from build123d import *

# Parameters (mm, degrees)
SKETCH1_R           = 2.5527
BOSS_EXTRUDE1_DEPTH = 2.54
SKETCH7_W           = 88.9
SKETCH7_H           = 19.05
BOSS_EXTRUDE2_DEPTH = 2.54
SKETCH6_W           = 38.1
SKETCH6_H           = 2.54
SKETCH6_W_2         = 2.54
SKETCH6_H_2         = 12.7
BOSS_EXTRUDE3_DEPTH = 16.51
CUT_EXTRUDE1_DEPTH  = 3.54


with BuildPart() as part:
    # Sketch1 → Boss-Extrude1 (new body)
    with BuildSketch(Plane(origin=(0, 0, 0), x_dir=(1, 0, 0), z_dir=(0, 1, 0))):
        with BuildLine():
            Line((44.45, -20.3835), (-44.45, -20.3835))
            Line((-44.45, -20.3835), (-44.45, 20.3835))
            Line((-44.45, 20.3835), (-35.2425, 20.3835))
            ThreePointArc((-35.2425, 20.3835), (-32.99743597, 19.45356403), (-32.0675, 17.2085))
            Line((-32.0675, 17.2085), (-32.0675, 1.3335))
            Line((-32.0675, 1.3335), (32.0675, 1.3335))
            Line((32.0675, 1.3335), (32.0675, 17.2085))
            ThreePointArc((32.0675, 17.2085), (32.99743597, 19.45356403), (35.2425, 20.3835))
            Line((35.2425, 20.3835), (44.45, 20.3835))
            Line((44.45, 20.3835), (44.45, -20.3835))
        make_face()
        with Locations((37.1475, -14.0335)):
            Circle(SKETCH1_R, mode=Mode.SUBTRACT)
        with Locations((37.1475, 14.0335)):
            Circle(SKETCH1_R, mode=Mode.SUBTRACT)
        with Locations((-37.1475, -14.0335)):
            Circle(SKETCH1_R, mode=Mode.SUBTRACT)
        with Locations((-37.1475, 14.0335)):
            Circle(SKETCH1_R, mode=Mode.SUBTRACT)
    extrude(amount=BOSS_EXTRUDE1_DEPTH)

    # Sketch7 → Boss-Extrude2 (add)
    with BuildSketch(Plane(origin=(0, 2.54, 0), x_dir=(1, 0, 0), z_dir=(0, 1, 0))):
        with Locations((0, -29.9085)):
            Rectangle(SKETCH7_W, SKETCH7_H)
    extrude(amount=-BOSS_EXTRUDE2_DEPTH)

    # Sketch6 → Boss-Extrude3 (add)
    with BuildSketch(Plane(origin=(0, 0, 0), x_dir=(-1, 0, 0), z_dir=(0, -1, 0))):
        with Locations((0, -36.195)):
            Rectangle(SKETCH6_W, SKETCH6_H)
        with Locations((0, -1.905)):
            Rectangle(SKETCH6_W, SKETCH6_H)
        with Locations((27.94, -19.05)):
            Rectangle(SKETCH6_W_2, SKETCH6_H_2)
        with Locations((-27.94, -19.05)):
            Rectangle(SKETCH6_W_2, SKETCH6_H_2)
    extrude(amount=BOSS_EXTRUDE3_DEPTH)

    # Sketch8 → Cut-Extrude1 (cut, through all)
    with BuildSketch(Plane.XZ):
        with BuildLine():
            Line((-44.45, 39.4335), (-31.75, 39.4335))
            Line((-31.75, 39.4335), (-31.75, 23.5585))
            ThreePointArc((-31.75, 23.5585), (-32.67993597, 21.31343597), (-34.925, 20.3835))
            Line((-34.925, 20.3835), (-44.45, 20.3835))
            Line((-44.45, 20.3835), (-44.45, 39.4335))
        make_face()
        with BuildLine():
            Line((44.45, 20.3835), (34.925, 20.3835))
            ThreePointArc((34.925, 20.3835), (32.67993597, 21.31343597), (31.75, 23.5585))
            Line((31.75, 23.5585), (31.75, 39.4335))
            Line((31.75, 39.4335), (44.45, 39.4335))
            Line((44.45, 39.4335), (44.45, 20.3835))
        make_face()
    extrude(amount=-CUT_EXTRUDE1_DEPTH, mode=Mode.SUBTRACT)


solid = part.part
Input: part model. Units: mm. Frame: model coordinates. A direction names the side the tool comes from. Coordinates: 2 decimals unless noted, no trailing zeros. Order: outer loops, then holes, each group sorted by start corner. A loop starts at its lowest first (then second) coordinate and runs counter-clockwise, first axis right, second up. Notation, with made-up numbers: M 45.25,57 L 92.25,57 A13 ccw 92.25,81 Z; hole C 12,5 d5. An arc over 180 degrees is marked long. Answer in a Markdown table with one row per item.
(1) Section query A-A, the plane y = -9.25. Output: boundary loops of the cut face in (x, z) (3 decimals), plus the area to 3 significant figures.
Numbers:
| item | result |
|---|---|
| outline | M -29.21,12.7 L -26.67,12.7 L -26.67,25.4 L -29.21,25.4 Z; M -19.05,0.635 L 19.05,0.635 L 19.05,3.175 L -19.05,3.175 Z; M -19.05,34.925 L 19.05,34.925 L 19.05,37.465 L -19.05,37.465 Z; M 26.67,12.7 L 29.21,12.7 L 29.21,25.4 L 26.67,25.4 Z |
| area | 258 mm^2 |
(2) Access query for faces 4 (the flat face through (-28, -8, 12.7)), 5 (the flat face through (-29.21, -8, 19)), 6 (the flat face through (-26.67, -8, 19)), 7 (the flat face through (-31.75, 1, 32)), 8 (the flat face through (19.05, -8, 2)). Directions: +Z, -Z, +X, -X, +Y, -Y. A direction counts if a zero-diameter tool reaches every point of the face in a straight line with its end or side. Return the directions, or none.
Numbers:
| item | result |
|---|---|
| face 4 | -Z, +X, -X, -Y |
| face 5 | +Z, -Z, -X, -Y |
| face 6 | +Z, -Z, -Y |
| face 7 | +Z, -X, +Y, -Y |
| face 8 | +Z, -Z, +X, -Y |
(3) Contact query for flat-ended pins moving along their axis: pin 1 Ø0.8 at (x, y) = (-42, 2) entering from +Z; pin 2 Ø4 at (y, z) = (-5, 18.5) entering from -X; pin 3 Ø0.8 at (y, z) = (-7, 2) entering from -X; pin 4 Ø5 at (y, z) = (-13, 29) entering from -X. Output: stop coordinate, or through.
Numbers:
| item | result |
|---|---|
| pin 1 | stops at z = 20.38 |
| pin 2 | stops at x = -29.21 |
| pin 3 | stops at x = -19.05 |
| pin 4 | passes through |
(4) Material intervals for line 1 (X direction, y = -11.75, z = 19); line 2 (Z direction, x = 13, y = -2.75) (3 decimals); line 3 (Z direction, x = 21, y = 0.75), sorted ascending. Write a range as [from, to].
Numbers:
| item | result |
|---|---|
| line 1 | x = [-29.21, -26.67], [26.67, 29.21] |
| line 2 | z = [0.635, 3.175], [34.925, 37.465] |
| line 3 | z = [-1.33, 39.43] |
(5) Section query C-C, the plane x = -18. Output: boundary loops of the cut face in (y, z) (1 decimal), plus the area to 3 significant figures.
Numbers:
| item | result |
|---|---|
| outline | M -16.5,0.6 L 0,0.6 L 0,-1.3 L 2.5,-1.3 L 2.5,39.4 L 0,39.4 L 0,37.5 L -16.5,37.5 L -16.5,34.9 L 0,34.9 L 0,3.2 L -16.5,3.2 Z |
| area | 187 mm^2 |
(6) Section query D-D, the plane z = 15. Output: boundary loops of the cut face in (x, y).
Numbers:
| item | result |
|---|---|
| outline | M -44.45,0 L -39.51,0 L -39.51,2.54 L -44.45,2.54 Z; M -34.78,0 L -29.21,0 L -29.21,-16.51 L -26.67,-16.51 L -26.67,0 L 26.67,0 L 26.67,-16.51 L 29.21,-16.51 L 29.21,0 L 34.78,0 L 34.78,2.54 L -34.78,2.54 Z; M 39.51,0 L 44.45,0 L 44.45,2.54 L 39.51,2.54 Z |
(7) Section query B-B, the plane z = -9. Output: boundary loops of the cut face in (x, y), plus the area to 3 significant figures.
Numbers:
| item | result |
|---|---|
| outline | M -44.45,0 L -32.07,0 L -32.07,2.54 L -44.45,2.54 Z; M 32.07,0 L 44.45,0 L 44.45,2.54 L 32.07,2.54 Z |
| area | 62.9 mm^2 |
(8) Draft query along Z for faces 1 (the cylindrical face through (-34.71, 1.25, 13.27)), 2 (the flat face through (-19.05, -8, 36)), 3 (the flat face through (-40, 1, -20.384)). Return one class per face: pulls with the +Z half, pulls with the -Z half, needs draft (parallel to the pull), parting line crosses it, or undercut.
Numbers:
| item | result |
|---|---|
| face 1 | undercut |
| face 2 | needs draft |
| face 3 | pulls with the -Z half |
